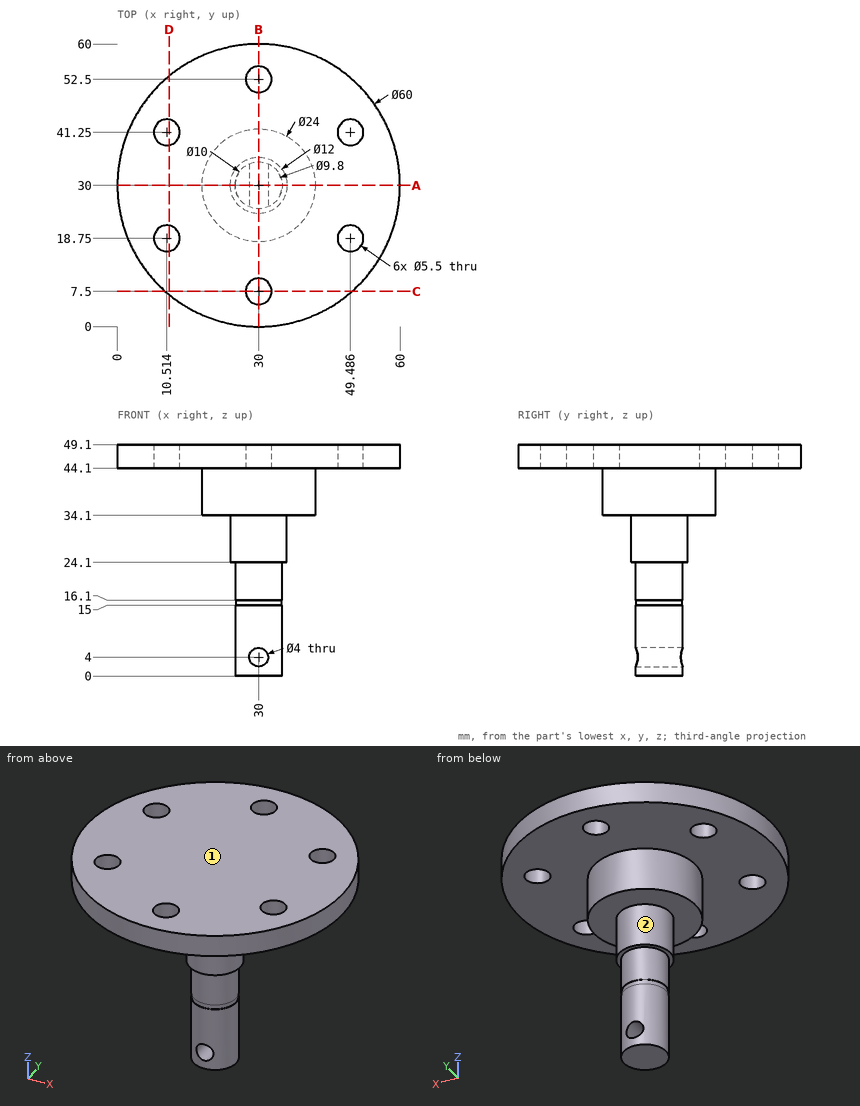
Geometry: see drawing. Coordinates: mm, zero at the bounding-box minimum. A direction names the side the tool comes from. Round coordinates to 2 decimals unless told otherwise and drop trailing zeros. Write each loop counter-clockwise with the first axis right and the second up, starting at its lowest first coordinate (ties: lowest second). Pieces come first, ordered by that corner, then holes.
Item 1: Material intervals for L1, parallel to Y at x = 30, z = 47; L2, parallel to Z at x = 30, y = 28; L3, parallel to Y at x = 28, z = 46 (1 decimal), sorted ascending.
Item 2: Pin query (flat end, axial travel): P1, Ø5, axis at x = 26.5, z = 43.5, coming from the +Y side; P2, Ø2, axis at x = 21.5, y = 21, coming from the -Z side; P3, Ø1.5, axis at x = 26, y = 48.5, coming from the -Z side. Return the tip coordinate at first contact, or that it passes through.
Item 3: Section query B-B (x = 30). Give the number of separate pieces and of enclosed holes in the cut face, plus the area to 3 significant figures.
Item 4: Set-up query: the marked faces 1 and 2. Return all of +Z, -Z, +X, -X, +Y, -Y with unobstructed straight access to the full face (end or side cutting, diameter ignored); none if empty.
Item 5: Section query C-C (y = 7.5). Return loops of the section in (x, z).
Item 6: Section query A-A (y = 30). Return loops of the section in (x, z), plus the area to 3 significant figures.
Item 7: Section query D-D (x = 11). Return loops of the section in (y, z), plus the area to 3 significant figures.
Completed:
1. L1: y = 0 to 4.75, 10.25 to 49.75, 55.25 to 60
1. L2: z = 0 to 2, 6 to 49.1
1. L3: y = 0.1 to 5.6, 9.4 to 50.6, 54.4 to 59.9
2. P1: stops at y = 59.98
2. P2: stops at z = 34.1
2. P3: stops at z = 44.1
3. separate pieces: 4
3. enclosed holes: 0
3. area: 806 mm2
4. face 1: +Z, +X, -X, +Y, -Y
4. face 2: -Z
5. outline: (10.16, 44.1) - (27.25, 44.1) - (27.25, 49.1) - (10.16, 49.1) - close; (32.75, 44.1) - (49.84, 44.1) - (49.84, 49.1) - (32.75, 49.1) - close
6. outline: (0, 44.1) - (18, 44.1) - (18, 34.1) - (24, 34.1) - (24, 24.1) - (25, 24.1) - (25, 16.1) - (25.1, 16.1) - (25.1, 15) - (25, 15) - (25, 0) - (35, 0) - (35, 15) - (34.9, 15) - (34.9, 16.1) - (35, 16.1) - (35, 24.1) - (36, 24.1) - (36, 34.1) - (42, 34.1) - (42, 44.1) - (60, 44.1) - (60, 49.1) - (0, 49.1) - close; hole circle Ø4 at (30, 4)
6. area: 888 mm2
7. outline: (6.78, 44.1) - (16.04, 44.1) - (16.04, 49.1) - (6.78, 49.1) - close; (21.46, 44.1) - (38.54, 44.1) - (38.54, 49.1) - (21.46, 49.1) - close; (43.96, 44.1) - (53.22, 44.1) - (53.22, 49.1) - (43.96, 49.1) - close
7. area: 178 mm2
